Could you check a few things on this model? Use its own coordinates, in mm. A direction names the side the tool comes from. Give positions to 0.01 mm unless a question says otherwise; leave off trailing zeros. Loops run counter-clockwise (first coordinate to the right, second up) from the corner with the lowest first, then second, coordinate; pieces in that order, holes last.
1. I need wall thicknesses on line 1 along Z through (x, y) = (108, 7.5); line 2 along X through (y, z) = (4.25, -12); line 3 along X through (y, z) = (5.25, -14.5). Which ranges of each line are inside material? Lowest first, please.
2. Imagine slicing it at A-A (y = 4.25). List the corners of the cut face in (x, z) for me.
3. For faces 1 (the flat face through (86, 2, -35)), 2 (the flat face through (16, 0, -37)), 3 (the flat face through (17, 10, -37)), 4 (the flat face through (85, 11, -35)), which set-ups out of +Z, -Z, +X, -X, +Y, -Y let a thin tool reach every point of the face, with its end or its side?
4. Imagine slicing it at B-B (z = -53.5). List the corners of the cut face in (x, y) for me, plus the area to 3 significant figures.
5. Thinking about a two-plate mould opening in X: for faces 5 (the cylindrical face through (102.905, 4.93, -12.224)), 6 (the flat face through (35, 11, -35)), 7 (the flat face through (104, 0, -37)), which applies, +X half, -X half, draft (parallel to the pull), parting line (faces both ways), or undercut?
6. Imagine slicing it at C-C (z = -10). List the corners of the cut face in (x, y) for me.
7. Imagine slicing it at D-D (x = 61.5). List the corners of the cut face in (y, z) for me, plus the area to 3 significant figures.
8. For P1, Ø5, axis at x = 12.5, z = -50, coming from the +Y side; P2, Ø6, axis at x = 48.5, z = -42, coming from the -Y side; P3, Ø0.9, axis at y = 11, z = -25, coming from the -X side, each with a flat end and sliding along its axis, tell me the tip position at first contact or that it passes through.
```python
from build123d import *

# Parameters (mm, degrees)
SKETCH1_R           = 5.1
SKETCH1_W           = 50
SKETCH1_H           = 72
BOSS_EXTRUDE7_DEPTH = 10
CUT_EXTRUDE2_DEPTH  = 72
SKETCH7_W           = 50
SKETCH7_H           = 72
BOSS_EXTRUDE8_DEPTH = 3


with BuildPart() as part:
    # Sketch1 → Boss-Extrude7 (new body)
    with BuildSketch(Plane(origin=(0, 0, 0), x_dir=(1, 0, 0), z_dir=(0, 1, 0))):
        with BuildLine():
            ThreePointArc((0, 12), (3.514718626, 3.514718626), (12, 0))
            Line((12, 0), (35, 0))
            Line((35, 0), (35, 72))
            Line((35, 72), (12, 72))
            ThreePointArc((12, 72), (3.514718626, 68.485281374), (0, 60))
            Line((0, 60), (0, 12))
        make_face()
        with Locations((12, 12)):
            Circle(SKETCH1_R, mode=Mode.SUBTRACT)
        with Locations((12, 60)):
            Circle(SKETCH1_R, mode=Mode.SUBTRACT)
        with Locations((60, 36)):
            Rectangle(SKETCH1_W, SKETCH1_H)
        with BuildLine():
            Line((85, 72), (85, 0))
            Line((85, 0), (108, 0))
            ThreePointArc((108, 0), (116.485281374, 3.514718626), (120, 12))
            Line((120, 12), (120, 60))
            ThreePointArc((120, 60), (116.485281374, 68.485281374), (108, 72))
            Line((108, 72), (85, 72))
        make_face()
        with Locations((108, 12)):
            Circle(SKETCH1_R, mode=Mode.SUBTRACT)
        with Locations((108, 60)):
            Circle(SKETCH1_R, mode=Mode.SUBTRACT)
    extrude(amount=BOSS_EXTRUDE7_DEPTH)

    # Sketch5 → Cut-Extrude2 (cut)
    with BuildSketch(Plane.XY):
        Polygon((32, 0), (35, 3), (85, 3), (88, 0), align=None)
    extrude(amount=-CUT_EXTRUDE2_DEPTH, mode=Mode.SUBTRACT)

    # Sketch7 → Boss-Extrude8 (add)
    with BuildSketch(Plane(origin=(0, 10, 0), x_dir=(1, 0, 0), z_dir=(0, 1, 0))):
        with Locations((60, 36)):
            Rectangle(SKETCH7_W, SKETCH7_H)
    extrude(amount=BOSS_EXTRUDE8_DEPTH)


solid = part.part
```
Derived:
1. line 1: z = -72 to -65.1, -54.9 to -17.1, -6.9 to 0
1. line 2: x = 0 to 6.9, 17.1 to 102.9, 113.1 to 120
1. line 3: x = 0 to 7.55, 16.45 to 103.55, 112.45 to 120
2. outline: (0, -60) arc R12 ccw to (12, -72) - (108, -72) arc R12 ccw to (120, -60) - (120, -12) arc R12 ccw to (108, 0) - (12, 0) arc R12 ccw to (0, -12) - close; hole circle Ø10.2 at (12, -60); hole circle Ø10.2 at (12, -12); hole circle Ø10.2 at (108, -60); hole circle Ø10.2 at (108, -12)
3. face 1: +Z, -Z, -Y
3. face 2: +Z, -Z, +X, -X, -Y
3. face 3: +Z, -Z, -X, +Y
3. face 4: +Z, -Z, +X, +Y
4. outline: (0, 0) - (32, 0) - (35, 3) - (85, 3) - (88, 0) - (120, 0) - (120, 10) - (85, 10) - (85, 13) - (35, 13) - (35, 10) - (0, 10) - close
4. area: 1,190 mm2
5. face 5: undercut
5. face 6: -X half
5. face 7: draft
6. outline: (0.17, 0) - (7.31, 0) - (7.31, 10) - (0.17, 10) - close; (16.69, 0) - (32, 0) - (35, 3) - (85, 3) - (88, 0) - (103.31, 0) - (103.31, 10) - (85, 10) - (85, 13) - (35, 13) - (35, 10) - (16.69, 10) - close; (112.69, 0) - (119.83, 0) - (119.83, 10) - (112.69, 10) - close
7. outline: (3, -72) - (13, -72) - (13, 0) - (3, 0) - close
7. area: 720 mm2
8. P1: stops at y = 10
8. P2: stops at y = 3
8. P3: stops at x = 35
